```python
from build123d import *

# Parameters (mm, degrees)
F0_W     = 40.2463
F0_H     = 43.4848
F1_DEPTH = 1.524
F2_W     = 40.2463
F2_H     = 14.097
F3_DEPTH = 1.524
F4_R     = 3.175
F5_DEPTH = 25.4


with BuildPart() as f1:
    # F0 (on Top) → F1 (new body)
    with BuildSketch(Plane.XY):
        Rectangle(F0_W, F0_H)
    extrude(amount=F1_DEPTH)

    # F2 (on face) → F3 (join)
    with BuildSketch(Plane.XZ.offset(21.7424)):
        with Locations((0, 3.4925)):
            Rectangle(F2_W, F2_H)
    extrude(amount=F3_DEPTH)

    # F4 (on face) → F5 (cut)
    with BuildSketch(Plane.XY.offset(1.524)):
        with Locations((15.04315, 15.748)):
            Circle(F4_R)
        with Locations((15.04315, -9.8552)):
            Circle(F4_R)
        with Locations((-15.04315, 15.748)):
            Circle(F4_R)
        with Locations((-15.04315, -9.8552)):
            Circle(F4_R)
    extrude(amount=-F5_DEPTH, mode=Mode.SUBTRACT)


solid = f1.part
```
CAD build for the part. Positions are in the model's coordinates, mm. A direction names the side the tool comes from. Coordinates: 2 decimals unless noted, no trailing zeros. Write each loop counter-clockwise with the first axis right and the second up, starting at its lowest first coordinate (ties: lowest second). Pieces come first, ordered by that corner, then holes. Notation, with made-up numbers: (31.25, 68.25) -> (71.25, 68.25) arc R26 ccw to (71.25, 97.25) -> close; hole circle Ø4 at (9.5, 89). An arc over 180 degrees is marked (long way). Return JSON: item names as keys, results as strings. Group by question number.
Q1. Drill centre lines: line 1 (Z direction, x = -4, y = 13); line 2 (Y direction, x = -9, z = 6.5). Where is each one in solid material? Low to high.
Q2. Cut at D-D, the plane y = -4. Give the cut face in (x, z), then the cut area to 3 significant figures.
Q3. Cut at C-C, the plane z = 0.5. Give the cut face in (x, y) (3 decimals), then the cut area to 3 significant figures.
Q4. Cut at A-A, the plane y = -10.5. Give the cut face in (x, z), then the cut area to 3 significant figures.
Q5. Which spindle directions (+Z, -Z, +X, -X, +Y, -Y) get a long thin tool onto all of the face, cutting with end or side? Do faces 1 (the face through (0, 0, 1.524)), 2 (the face through (20.123, -6, 1)), 3 (the face through (0, -21.742, -2)). Say none if no direction does.
Q6. Flat gauge pins, fed straight in: pin 1 (7 mm diameter, centred on x = 4.5, z = 8, fed in from +Y); pin 2 (7.5 mm diameter, centred on x = 15.04, y = -9.86, fed in from -Z); pin 3 (10 mm diameter, centred on x = -15.04, y = 15.75, fed in from +Z); pin 4 (8 mm diameter, centred on y = -6, z = -1, fed in from -X). Where does each tip first touch, or does it go through?
Q7. Cut at B-B, the plane x = 4.5. Give the cut face in (y, z).
Q8. Pull direction Y, two halves, no side cores. Call faces 4 (the face through (0, -23.266, 4)), 5 (the face through (0, 0, 0)), 6 (the face through (0, -21.742, 6)), 7 (the face through (-17.56, -11.79, 0.77)): released by +Y, released by -Y, zero draft, split by the parting line, or undercut.
Returned:
{
 "1": {"line 1": "z = 0 to 1.52", "line 2": "y = -23.27 to -21.74"},
 "2": {"outline": "(-20.12, 0) -> (20.12, 0) -> (20.12, 1.52) -> (-20.12, 1.52) -> close", "area": "61.3 mm2"},
 "3": {"outline": "(-20.123, -23.266) -> (20.123, -23.266) -> (20.123, 21.742) -> (-20.123, 21.742) -> close; hole circle Ø6.35 at (-15.043, -9.855); hole circle Ø6.35 at (-15.043, 15.748); hole circle Ø6.35 at (15.043, -9.855); hole circle Ø6.35 at (15.043, 15.748)", "area": "1,680 mm2"},
 "4": {"outline": "(-20.12, 0) -> (-18.15, 0) -> (-18.15, 1.52) -> (-20.12, 1.52) -> close; (-11.93, 0) -> (11.93, 0) -> (11.93, 1.52) -> (-11.93, 1.52) -> close; (18.15, 0) -> (20.12, 0) -> (20.12, 1.52) -> (18.15, 1.52) -> close", "area": "42.4 mm2"},
 "5": {"face 1": "+Z, +X, -X, +Y", "face 2": "+Z, -Z, +X, +Y, -Y", "face 3": "-Z, +X, -X, +Y"},
 "6": {"pin 1": "stops at y = -21.74", "pin 2": "stops at z = 0", "pin 3": "stops at z = 1.52", "pin 4": "stops at x = -20.12"},
 "7": {"outline": "(-23.27, -3.56) -> (-21.74, -3.56) -> (-21.74, 0) -> (21.74, 0) -> (21.74, 1.52) -> (-21.74, 1.52) -> (-21.74, 10.54) -> (-23.27, 10.54) -> close"},
 "8": {"face 4": "released by -Y", "face 5": "zero draft", "face 6": "released by +Y", "face 7": "undercut"}
}
